The model under review builds one solid part; all positions refer to its coordinate system, in mm. Round coordinates to 2 decimals unless told otherwise and drop trailing zeros. Order: outer loops, then holes, each group sorted by start corner. A loop starts at its lowest first (then second) coordinate and runs counter-clockwise, first axis right, second up. Notation, with made-up numbers: M 3.25,70.25 L 13.25,70.25 A19 cw 13.25,103.25 Z; hole C 72,77.5 d10. An arc over 180 degrees is marked long. Answer as a JSON object with one key per item and string values. Group by question number.
1) Consider section B-B, the plane x = 0. Write out the cut boundary in (y, z) (3 decimals), then the cut area to 3 significant figures.
2) To check wall thickness, follow line 1 (X direction, y = 0.2, z = 0); line 2 (Z direction, x = -19, y = -2). State the ranges of each line that lie inside material, in increasing order.
3) Consider section A-A, the plane z = 0. Write out the cut boundary in (x, y) (3 decimals).
4) Consider section C-C, the plane y = 0.25. Write out the cut boundary in (x, z), then the cut area to 3 significant figures.
5) Insertion check: pin 1 Ø1.5 at (x, y) = (19.5, 2) entering from -Z; pin 2 Ø6 at (x, z) = (28, 22) entering from +Y; pin 3 Ø4 at (y, z) = (-1.5, -7.5) entering from -X. Each pin has a flat end and moves straight along its axis. Give the tip position at first contact, or say it passes through.
6) The part is to be moulded in two halves that separate along Z. For faces 1 (the cylindrical face through (11.433, 0.024, 27.574)), 2 (the cylindrical face through (21.36, -0.02, -27.85)), say which applies: +Z half, -Z half, draft (parallel to the pull), parting line (faces both ways), or undercut.
```python
from build123d import *

# Parameters (mm, degrees)
F5_DEPTH = 6


# Not quite as in the source:
# - a feature of the source that left no trace in its solid (it failed there, or was rolled back) is left out


with BuildPart() as f1:
    # F0 (on Right) → F1 (revolve)
    with BuildSketch(Plane.YZ):
        with BuildLine():
            ThreePointArc((1.75, 29.85), (4.375, 32.475), (1.75, 35.1))
            Line((1.75, 35.1), (-1.75, 35.1))
            ThreePointArc((-1.75, 35.1), (-4.375, 32.475), (-1.75, 29.85))
            Line((-1.75, 29.85), (1.75, 29.85))
        make_face()
    revolve(axis=Axis((0, -4.6846177429, 0), (0, -1, 0)))


with BuildPart() as f3:
    # F2 (on Right) → F3 (revolve)
    with BuildSketch(Plane.YZ):
        with BuildLine():
            ThreePointArc((4.3570501582, 32.1685453172), (3.4944456795, 30.5134867395), (1.75, 29.85))
            Line((1.75, 29.85), (-1.75, 29.85))
            ThreePointArc((-1.75, 29.85), (-3.6061553006, 30.6188446994), (-4.375, 32.475))
            Line((-4.375, 32.475), (-4.375, 27.1685775369))
            Line((-4.375, 27.1685775369), (4.375, 27.1685775369))
            Line((4.375, 27.1685775369), (4.3570501582, 32.1685453172))
        make_face()
    revolve(axis=Axis((0, -6.0206142662, 0), (0, -1, 0)))

    # F4 (on Front) → F5 (join, symmetric)
    with BuildSketch(Plane.XZ):
        with BuildLine():
            ThreePointArc((-0.8, -1.805720078), (-1.9541006025, -0.286558607), (-1.2847665158, 1.5))
            Line((-1.2847665158, 1.5), (1.2847665158, 1.5))
            ThreePointArc((1.2847665158, 1.5), (1.9541006025, -0.286558607), (0.8, -1.805720078))
            Line((0.8, -1.805720078), (0.8, -6.9541354603))
            ThreePointArc((0.8, -6.9541354603), (2.1957679989, -6.6466986463), (3.5, -6.0621778265))
            ThreePointArc((3.5, -6.0621778265), (3.694735219, -5.9454967548), (3.8855844605, -5.8225624428))
            ThreePointArc((3.8855844605, -5.8225624428), (3.8880716888, -5.8324992461), (3.890563158, -5.8424349868))
            ThreePointArc((3.890563158, -5.8424349868), (8.500978981, -15.0837914383), (16.568096168, -21.5320643401))
            ThreePointArc((16.568096168, -21.5320643401), (18.1794560768, -20.1900713752), (19.6825117076, -18.727795873))
            ThreePointArc((19.6825117076, -18.727795873), (11.7812454852, -13.0384635672), (7.4660124048, -4.3105042717))
            ThreePointArc((7.4660124048, -4.3105042717), (17.1822634181, -3.6836260948), (26.0600028367, -7.6816572125))
            ThreePointArc((26.0600028367, -7.6816572125), (26.5748427535, -5.6488351019), (26.9313627985, -3.5823600038))
            ThreePointArc((26.9313627985, -3.5823600038), (17.3134360615, 0.1798319646), (7.0049786976, -0.4481090365))
            ThreePointArc((7.0049786976, -0.4481090365), (6.9951283591, -0.4509192312), (6.9852792208, -0.4537336299))
            ThreePointArc((6.9852792208, -0.4537336299), (6.9963188373, -0.2269861825), (7, 0))
            ThreePointArc((7, 0), (6.0621778265, 3.5), (3.5, 6.0621778265))
            ThreePointArc((3.5, 6.0621778265), (3.3015836183, 6.1724829373), (3.0996947604, 6.2762960727))
            ThreePointArc((3.0996947604, 6.2762960727), (3.1070566702, 6.2834184773), (3.1144155395, 6.2905440233))
            ThreePointArc((3.1144155395, 6.2905440233), (8.8124570805, 14.9039594738), (10.3632666305, 25.1144243439))
            ThreePointArc((10.3632666305, 25.1144243439), (8.3953866767, 25.838906477), (6.3774911291, 26.4094530856))
            ThreePointArc((6.3774911291, 26.4094530856), (5.4010179329, 16.722089662), (0, 8.6210085433))
            ThreePointArc((0, 8.6210085433), (-5.4010179329, 16.722089662), (-6.3774911291, 26.4094530856))
            ThreePointArc((-6.3774911291, 26.4094530856), (-8.3953866767, 25.838906477), (-10.3632666305, 25.1144243439))
            ThreePointArc((-10.3632666305, 25.1144243439), (-8.8124570805, 14.9039594738), (-3.1144155395, 6.2905440233))
            ThreePointArc((-3.1144155395, 6.2905440233), (-3.1070566702, 6.2834184773), (-3.0996947604, 6.2762960727))
            ThreePointArc((-3.0996947604, 6.2762960727), (-3.3015836183, 6.1724829373), (-3.5, 6.0621778265))
            ThreePointArc((-3.5, 6.0621778265), (-6.0621778265, 3.5), (-7, 0))
            ThreePointArc((-7, 0), (-6.9963188373, -0.2269861825), (-6.9852792208, -0.4537336299))
            ThreePointArc((-6.9852792208, -0.4537336299), (-6.9951283591, -0.4509192312), (-7.0049786976, -0.4481090365))
            ThreePointArc((-7.0049786976, -0.4481090365), (-17.3134360615, 0.1798319646), (-26.9313627985, -3.5823600038))
            ThreePointArc((-26.9313627985, -3.5823600038), (-26.5748427535, -5.6488351019), (-26.0600028367, -7.6816572125))
            ThreePointArc((-26.0600028367, -7.6816572125), (-17.1822634181, -3.6836260948), (-7.4660124048, -4.3105042717))
            ThreePointArc((-7.4660124048, -4.3105042717), (-11.7812454852, -13.0384635672), (-19.6825117076, -18.727795873))
            ThreePointArc((-19.6825117076, -18.727795873), (-18.1794560768, -20.1900713752), (-16.568096168, -21.5320643401))
            ThreePointArc((-16.568096168, -21.5320643401), (-8.500978981, -15.0837914383), (-3.890563158, -5.8424349868))
            ThreePointArc((-3.890563158, -5.8424349868), (-3.8880716888, -5.8324992461), (-3.8855844605, -5.8225624428))
            ThreePointArc((-3.8855844605, -5.8225624428), (-3.694735219, -5.9454967548), (-3.5, -6.0621778265))
            ThreePointArc((-3.5, -6.0621778265), (-2.1957679989, -6.6466986463), (-0.8, -6.9541354603))
            Line((-0.8, -6.9541354603), (-0.8, -1.805720078))
        make_face()
    extrude(amount=F5_DEPTH, both=True)

    # F6 (on Right) → F7 (revolve, cut)
    with BuildSketch(Plane.YZ):
        with BuildLine():
            Line((-13.0535820499, 2.701601783), (-6, 4))
            ThreePointArc((-6, 4), (-1.8810208663, 15.3523786055), (-4.375, 27.1685775369))
            Line((-4.375, 27.1685775369), (-11.726167053, 27.1685775369))
            Line((-11.726167053, 27.1685775369), (-13.0535820499, 2.701601783))
        make_face()
        with BuildLine():
            Line((12.8782450573, 27.7328483518), (4.375, 27.1685775369))
            ThreePointArc((4.375, 27.1685775369), (1.8810208663, 15.3523786055), (6, 4))
            Line((6, 4), (14.3638671536, 5.3453556511))
            Line((14.3638671536, 5.3453556511), (12.8782450573, 27.7328483518))
        make_face()
    revolve(axis=Axis((0, -4.9612242728, 0), (0, 1, 0)), mode=Mode.SUBTRACT)


solid = f1.part
```
Results list:
{
 "1": {"outline": "M -1.75,-35.1 L 1.75,-35.1 A2.625 ccw 1.75,-29.85 L -1.75,-29.85 A2.625 ccw Z; M -1.75,29.85 L 1.75,29.85 A2.625 ccw 1.75,35.1 L -1.75,35.1 A2.625 ccw Z", "area": "80.0 mm^2"},
 "2": {"line 1": "-35.1 to -29.85, 29.85 to 35.1", "line 2": "-29.5 to -23.04, 23.04 to 29.5"},
 "3": {"outline": "M -35.1,-1.75 A2.625 ccw -29.85,-1.75 L -29.85,1.75 A2.625 ccw -35.1,1.75 Z; M 29.85,-1.75 A2.625 ccw 35.1,-1.75 L 35.1,1.75 A2.625 ccw 29.85,1.75 Z"},
 "4": {"outline": "C 0,0 d70.2; hole C 0,0 d59.7", "area": "1,070 mm^2"},
 "5": {"pin 1": "z = -29.66", "pin 2": "y = 4.37", "pin 3": "x = -34.67"},
 "6": {"face 1": "undercut", "face 2": "parting line"}
}
